```python
from build123d import *

# Parameters (mm, degrees)
EXTRUDE_1_DEPTH     = 5
SKETCH_2_W          = 53
SKETCH_2_H          = 3
EXTRUDE_2_DEPTH     = 3
SKETCH_3_W          = 53
SKETCH_3_H          = 50
EXTRUDE_3_DEPTH     = 3
SKETCH_4_W          = 3
SKETCH_4_H          = 50
EXTRUDE_4_DEPTH     = 18
SKETCH_5_W          = 7
SKETCH_5_H          = 17.5
CUT_EXTRUDE_1_DEPTH = 3
SKETCH_7_W          = 12.5
SKETCH_7_H          = 19.5
CUT_EXTRUDE_2_DEPTH = 3


with BuildPart() as part:
    # Эскиз1 → Бобышка-Вытянуть1 (new body)
    with BuildSketch(Plane(origin=(0, 0, 0), x_dir=(1, 0, 0), z_dir=(0, 1, 0))):
        Polygon((2.25, 0), (-2.25, 0), (-4, 3), (4, 3), align=None)
    extrude(amount=EXTRUDE_1_DEPTH)

    # Эскиз2 → Бобышка-Вытянуть2 (add)
    with BuildSketch(Plane(origin=(0, 5, 0), x_dir=(1, 0, 0), z_dir=(0, 1, 0))):
        with Locations((0, 1.5)):
            Rectangle(SKETCH_2_W, SKETCH_2_H)
    extrude(amount=EXTRUDE_2_DEPTH)

    # Эскиз3 → Бобышка-Вытянуть3 (add)
    with BuildSketch(Plane.XY):
        with Locations((0, -17)):
            Rectangle(SKETCH_3_W, SKETCH_3_H)
    extrude(amount=EXTRUDE_3_DEPTH)

    # Эскиз4 → Бобышка-Вытянуть4 (add)
    with BuildSketch(Plane(origin=(26.5, 0, 0), x_dir=(0, 0, -1), z_dir=(1, 0, 0))):
        with Locations((-1.5, -17)):
            Rectangle(SKETCH_4_W, SKETCH_4_H)
    extrude(amount=EXTRUDE_4_DEPTH)

    # Эскиз5 → Вырез-Вытянуть1 (cut)
    with BuildSketch(Plane.XY.offset(3)):
        with Locations((-18, -5.75)):
            Rectangle(SKETCH_5_W, SKETCH_5_H)
        with Locations((-18, -28.25)):
            Rectangle(SKETCH_5_W, SKETCH_5_H)
        with Locations((6, -5.75)):
            Rectangle(SKETCH_5_W, SKETCH_5_H)
        with Locations((6, -28.25)):
            Rectangle(SKETCH_5_W, SKETCH_5_H)
        with Locations((-6, -5.75)):
            Rectangle(SKETCH_5_W, SKETCH_5_H)
        with Locations((-6, -28.25)):
            Rectangle(SKETCH_5_W, SKETCH_5_H)
        with Locations((30, -5.75)):
            Rectangle(SKETCH_5_W, SKETCH_5_H)
        with Locations((18, -5.75)):
            Rectangle(SKETCH_5_W, SKETCH_5_H)
        with Locations((18, -28.25)):
            Rectangle(SKETCH_5_W, SKETCH_5_H)
    extrude(amount=-CUT_EXTRUDE_1_DEPTH, mode=Mode.SUBTRACT)

    # Эскиз7 → Вырез-Вытянуть2 (cut)
    with BuildSketch(Plane.XY.offset(3)):
        with Locations((35.25, -29.25)):
            Rectangle(SKETCH_7_W, SKETCH_7_H)
    extrude(amount=-CUT_EXTRUDE_2_DEPTH, mode=Mode.SUBTRACT)


solid = part.part
```
The listing builds one solid part. Answer for the finished solid, in the listing's coordinates (mm). A direction names the side the tool comes from. Give positions to 0.01 mm unless a question says otherwise; leave off trailing zeros. Order: outer loops, then holes, each group sorted by start corner. A loop starts at its lowest first (then second) coordinate and runs counter-clockwise, first axis right, second up. Notation, with made-up numbers: (-6.5, -14.75) -> (46.5, -14.75) arc R8 cw to (46.5, -3.75) -> close; hole circle Ø3 at (6.25, -34.75). An arc over 180 degrees is marked (long way). Answer as a JSON object with one key per item and string values. Group by question number.
Item 1: The part is cut by section A-A on x = 19.5. Write down the section's boundary in (y, z).
Item 2: The part is cut by section D-D on z = -1.2. Write down the section's boundary in (x, y).
Item 3: The part is cut by section C-C on x = 36. Write down the section's boundary in (y, z), and give its area (3 significant figures).
Item 4: A tool of negligible diameter and unlimited length cuts with its end or side. For faces 1 (the flat face through (-18, -37, 2)), 2 (the flat face through (9, -17, 3)), from which of +Z, -Z, +X, -X, +Y, -Y can it reach the whole face along a straight path? Write none if from no direction.
Item 5: Determine the mould class of faces 3 (the flat face through (14.5, -28, 2)), 4 (the flat face through (-9.5, -28, 2)), 5 (the flat face through (-3.113, 2.465, -1.479)), 6 (the flat face through (0, 0, -2)) for opening direction X: pulls with the +X half, pulls with the -X half, needs draft (parallel to the pull), parting line crosses it, or undercut.
Item 6: The part is cut by section B-B on y = -25.5. Write down the section's boundary in (x, z), and give its area (3 significant figures).
Item 7: Consider L1, parallel to Y at x = 31, z = 0.2; L2, parallel to X at y = -32, z = 1.2; L3, parallel to X at y = -5.5, z = 0.4. Determine where each line is inside the solid, lowest interval first. Write a range as from..to.
Result set:
{
 "1": {"outline": "(-42, 0) -> (-37, 0) -> (-37, 3) -> (-42, 3) -> close; (-19.5, 0) -> (-14.5, 0) -> (-14.5, 3) -> (-19.5, 3) -> close; (3, 0) -> (5, 0) -> (5, -3) -> (8, -3) -> (8, 3) -> (3, 3) -> close"},
 "2": {"outline": "(-26.5, 5) -> (-2.95, 5) -> (-2.95, 0) -> (2.95, 0) -> (2.95, 5) -> (26.5, 5) -> (26.5, 8) -> (-26.5, 8) -> close"},
 "3": {"outline": "(-42, 0) -> (-39, 0) -> (-39, 3) -> (-42, 3) -> close; (-19.5, 0) -> (8, 0) -> (8, 3) -> (-19.5, 3) -> close", "area": "91.5 mm²"},
 "4": {"face 1": "+Z, -Z", "face 2": "+Z, +X, -X, +Y, -Y"},
 "5": {"face 3": "undercut", "face 4": "undercut", "face 5": "pulls with the -X half", "face 6": "needs draft"},
 "6": {"outline": "(-26.5, 0) -> (-21.5, 0) -> (-21.5, 3) -> (-26.5, 3) -> close; (-14.5, 0) -> (-9.5, 0) -> (-9.5, 3) -> (-14.5, 3) -> close; (-2.5, 0) -> (2.5, 0) -> (2.5, 3) -> (-2.5, 3) -> close; (9.5, 0) -> (14.5, 0) -> (14.5, 3) -> (9.5, 3) -> close; (21.5, 0) -> (29, 0) -> (29, 3) -> (21.5, 3) -> close; (41.5, 0) -> (44.5, 0) -> (44.5, 3) -> (41.5, 3) -> close", "area": "91.5 mm²"},
 "7": {"L1": "-42..-39, -19.5..-14.5, 3..8", "L2": "-26.5..-21.5, -14.5..-9.5, -2.5..2.5, 9.5..14.5, 21.5..29, 41.5..44.5", "L3": "-26.5..-21.5, -14.5..-9.5, -2.5..2.5, 9.5..14.5, 21.5..26.5, 33.5..44.5"}
}
